from build123d import *

# Parameters (mm, degrees)
BOSS_EXTRUDE1_REACH      = 130.098
BOSS_EXTRUDE1_END_RADIUS = 25
SKETCH2_R                = 4
SKETCH3_R                = 25
SKETCH3_R_2              = 20
BOSS_EXTRUDE2_DEPTH      = 50


with BuildPart() as part:
    # Sketch1 → Revolve1 (revolve)
    with BuildSketch(Plane(origin=(0, 0, 0), x_dir=(0, 0, -1), z_dir=(1, 0, 0)), mode=Mode.PRIVATE) as revolve1_sk:
        Polygon((22.320508076, 25), (100, 25), (100, 20), (20.980762114, 20), (0, 32.113248654), (0, 35), (5, 35), align=None)
    revolve(revolve1_sk.sketch.rotate(Axis((0, 0, 0), (0, 0, -1)), 90), axis=Axis((0, 0, 0), (0, 0, -1)))

    # Boss-Extrude1: up to this cylinder (the profile starts outside it)
    boss_extrude1_end = Plane(origin=(0, 0, -31.75833), z_dir=(0, 0, 1)) * Cylinder(BOSS_EXTRUDE1_END_RADIUS, 311.196, mode=Mode.PRIVATE)
    # Sketch2 → Boss-Extrude1 (add, up to the surface)
    with BuildSketch(Plane(origin=(0, 37, 0), x_dir=(1, 0, 0), z_dir=(0, 1, 0)), mode=Mode.PRIVATE) as boss_extrude1_sk1:
        with Locations(Location((0, 31.758330249, 0), (0, 0, 270))):
            Circle(SKETCH2_R)
    boss_extrude1_tool1 = extrude(boss_extrude1_sk1.sketch, amount=-BOSS_EXTRUDE1_REACH, mode=Mode.PRIVATE) - boss_extrude1_end
    boss_extrude1 = boss_extrude1_tool1.solids().sort_by_distance((0, 37, -31.75833))[0]
    add(boss_extrude1)

    # Mirror1: Boss-Extrude1 across plane
    add(boss_extrude1.mirror(Plane.ZX))

    # Sketch3 → Boss-Extrude2 (add)
    with BuildSketch(Plane(origin=(0, 0, -100), x_dir=(-1, 0, 0), z_dir=(0, 0, -1))):
        with Locations(Location((0, 0, 0), (0, 0, 180))):
            Circle(SKETCH3_R)
        with Locations(Location((0, 0, 0), (0, 0, 180))):
            Circle(SKETCH3_R_2, mode=Mode.SUBTRACT)
    extrude(amount=BOSS_EXTRUDE2_DEPTH)


solid = part.part
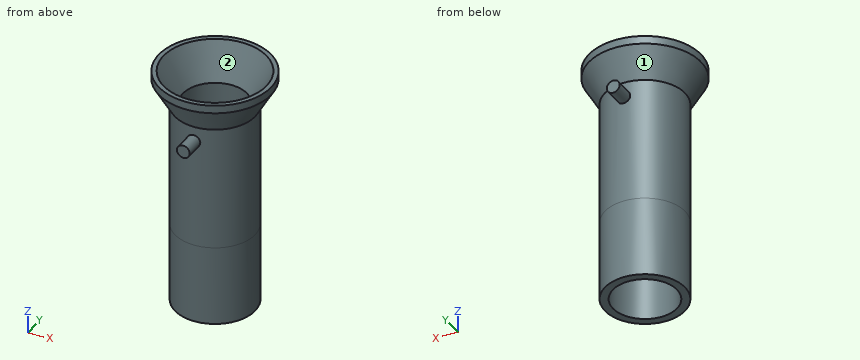
Work out the finished part from the listing and answer in its coordinate system (mm). Face numbers are marked on the shaded views. Give positions to 0.01 mm unless a question says otherwise; leave off trailing zeros. Order: outer loops, then holes, each group sorted by start corner. A loop starts at its lowest first (then second) coordinate and runs counter-clockwise, first axis right, second up. Notation, with made-up numbers: (6, 69.25) -> (16, 69.25) arc R20 ccw to (16, 74.25) -> close; hole circle Ø3 at (-13.75, 32). An arc over 180 degrees is marked (long way). Answer as a JSON object with one key per item and string values. Group by question number.
1. Section A-A on y = 0 is taken. Determine the outline of the cut face in (x, z), plus the area to 3 significant figures.
2. Section B-B on x = 0 is taken. Determine the outline of the cut face in (y, z), plus the area to 3 significant figures.
3. Section C-C on z = -138 is taken. Determine the outline of the cut face in (x, y).
4. Flat-ended cylindrical pins translate along their axes: pin 1 Ø12 at (y, z) = (-23, -24) entering from -X; pin 2 Ø2 at (y, z) = (1.5, -89.5) entering from +X (3 decimals); pin 3 Ø1 at (x, y) = (-2.5, -25.5) entering from +Z. Find the tip coordinate at first contact, or state that the pin passes through.
5. Consider line 1 along Y through (x, z) = (0, -123.5); line 2 along Y through (x, z) = (17, -62); line 3 along X through (y, z) = (13, -98.5). Determine where each line is inside the solid, lowest interval first. Write a range as [from, to].
6. The mould has two halves that part along Y. Classify the marked faces 1 and 2: released by +Y, released by -Y, zero draft, split by the parting line, or undercut.
Result sheet:
{
 "1": {"outline": "(-35, -5) -> (-25, -22.32) -> (-25, -150) -> (-20, -150) -> (-20, -20.98) -> (-32.11, 0) -> (-35, 0) -> close; (20, -150) -> (25, -150) -> (25, -22.32) -> (35, -5) -> (35, 0) -> (32.11, 0) -> (20, -20.98) -> close", "area": "1,520 mm^2"},
 "2": {"outline": "(-37, -35.76) -> (-25, -35.76) -> (-25, -150) -> (-20, -150) -> (-20, -20.98) -> (-32.11, 0) -> (-35, 0) -> (-35, -5) -> (-25, -22.32) -> (-25, -27.76) -> (-37, -27.76) -> close; (20, -150) -> (25, -150) -> (25, -35.76) -> (37, -35.76) -> (37, -27.76) -> (25, -27.76) -> (25, -22.32) -> (35, -5) -> (35, 0) -> (32.11, 0) -> (20, -20.98) -> close", "area": "1,710 mm^2"},
 "3": {"outline": "circle Ø50 at (0, 0); hole circle Ø40 at (0, 0)"},
 "4": {"pin 1": "stops at x = -18.73", "pin 2": "stops at x = 24.995", "pin 3": "stops at z = -10.38"},
 "5": {"line 1": "y = [-25, -20], [20, 25]", "line 2": "y = [-18.33, -10.54], [10.54, 18.33]", "line 3": "x = [-21.35, -15.2], [15.2, 21.35]"},
 "6": {"face 1": "split by the parting line", "face 2": "undercut"}
}
